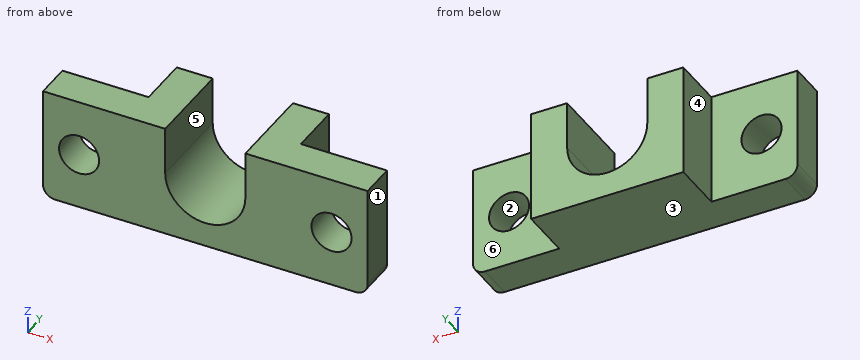
from build123d import *

# Parameters (mm, degrees)
SKETCH_1_W          = 81
SKETCH_1_H          = 28
EXTRUDE_1_DEPTH     = 9
SKETCH_2_W          = 38
SKETCH_2_H          = 28
EXTRUDE_2_DEPTH     = 13
CUT_EXTRUDE_1_DEPTH = 33
SKETCH_4_R          = 5
CUT_EXTRUDE_2_DEPTH = 33
SKETCH_5_R          = 5
CUT_EXTRUDE_3_DEPTH = 33
FILLET_1_R          = 3


with BuildPart() as part:
    # 스케치1 → 보스-돌출1 (new body)
    with BuildSketch(Plane(origin=(0, 0, 0), x_dir=(1, 0, 0), z_dir=(0, 1, 0))):
        with Locations((40.5, 14)):
            Rectangle(SKETCH_1_W, SKETCH_1_H)
    extrude(amount=EXTRUDE_1_DEPTH)

    # 스케치2 → 보스-돌출2 (add)
    with BuildSketch(Plane(origin=(0, 9, 0), x_dir=(1, 0, 0), z_dir=(0, 1, 0))):
        with Locations((40.5, 14)):
            Rectangle(SKETCH_2_W, SKETCH_2_H)
    extrude(amount=EXTRUDE_2_DEPTH)

    # 스케치3 → 컷-돌출1 (cut)
    with BuildSketch(Plane(origin=(0, 22, 0), x_dir=(1, 0, 0), z_dir=(0, 1, 0))):
        with BuildLine():
            Line((30.5, 0), (30.5, 11.914888689))
            ThreePointArc((30.5, 11.914888689), (40.5, 21.914888689), (50.5, 11.914888689))
            Line((50.5, 11.914888689), (50.5, 0))
            Line((50.5, 0), (30.5, 0))
        make_face()
    extrude(amount=-CUT_EXTRUDE_1_DEPTH, mode=Mode.SUBTRACT)

    # 스케치4 → 컷-돌출2 (cut)
    with BuildSketch(Plane(origin=(0, 9, 0), x_dir=(1, 0, 0), z_dir=(0, 1, 0))):
        with Locations(Location((9, 14, 0), (0, 0, 270))):
            Circle(SKETCH_4_R)
    extrude(amount=-CUT_EXTRUDE_2_DEPTH, mode=Mode.SUBTRACT)

    # 스케치5 → 컷-돌출3 (cut)
    with BuildSketch(Plane(origin=(0, 9, 0), x_dir=(1, 0, 0), z_dir=(0, 1, 0))):
        with Locations(Location((72, 14, 0), (0, 0, 270))):
            Circle(SKETCH_5_R)
    extrude(amount=-CUT_EXTRUDE_3_DEPTH, mode=Mode.SUBTRACT)

    # 필렛1
    fillet_1_edges = [part.edges().sort_by_distance(p)[0] for p in [
        (0, 4.5, -28),
        (81, 4.5, -28),
    ]]
    fillet(fillet_1_edges, radius=FILLET_1_R)


solid = part.part
Verification items for the finished model (mm, model axes). Face numbers are marked on the shaded views. A direction names the side the tool comes from. Give positions to 0.01 mm unless a question says otherwise; leave off trailing zeros. Write each loop counter-clockwise with the first axis right and the second up, starting at its lowest first coordinate (ties: lowest second). Pieces come first, ordered by that corner, then holes. Notation, with made-up numbers: (-17, 64.25) - (19, 64.25) arc R30 cw to (19, 89.25) - close; hole circle Ø7 at (71.5, 15). An arc over 180 degrees is marked (long way). Answer as CSV lines item,"result". Start each with the question number.
1. Thickness scan on line 1 (X direction, y = 7, z = -14); line 2 (Y direction, x = 15.5, z = -8); line 3 (X direction, y = 21.25, z = -8.25). Record the ranges inside material, lowest first.
2. Sectioned sample at C-C (z = -14). Record the boundary of the cut face in (x, y).
3. Sectioned sample at B-B (y = 3.25). Record the boundary of the cut face in (x, z).
4. Depth check by flat-ended pin: pin 1 (13 mm diameter, centred on y = 16.5, z = -8, fed in from +X); pin 2 (12 mm diameter, centred on x = 43, y = 15.5, fed in from +Z); pin 3 (4 mm diameter, centred on y = 15, z = -9.5, fed in from -X). Enter the tip coordinate at first touch or a pass-through.
5. Set-up check for the marked faces 4, 5 and 6: record each of +Z, -Z, +X, -X, +Y, -Y from which the full face is reachable in a straight line by a thin tool's end or side.
6. Sectioned sample at D-D (z = -5.5). Record the boundary of the cut face in (x, y), then the cut area to 3 significant figures.
7. Sectioned sample at A-A (x = 72). Record the boundary of the cut face in (y, z), then the cut area to 3 significant figures.
8. Draft check along X on the marked faces 1, 2 and 3. Enter one of: pulls with the +X half, pulls with the -X half, needs draft (parallel to the pull), parting line crosses it, or undercut.
Derived:
1,line 1,"0 to 4, 14 to 30.72, 50.28 to 67, 77 to 81"
1,line 2,"0 to 9"
1,line 3,"21.5 to 30.5, 50.5 to 59.5"
2,outline,"(0, 0) - (4, 0) - (4, 9) - (0, 9) - close; (14, 0) - (30.72, 0) - (30.72, 22) - (21.5, 22) - (21.5, 9) - (14, 9) - close; (50.28, 0) - (67, 0) - (67, 9) - (59.5, 9) - (59.5, 22) - (50.28, 22) - close; (77, 0) - (81, 0) - (81, 9) - (77, 9) - close"
3,outline,"(0, -25) arc R3 ccw to (3, -28) - (78, -28) arc R3 ccw to (81, -25) - (81, 0) - (50.5, 0) - (50.5, -11.91) arc R10 cw to (30.5, -11.91) - (30.5, 0) - (0, 0) - close; hole circle Ø10 at (9, -14); hole circle Ø10 at (72, -14)"
4,pin 1,"x = 59.5"
4,pin 2,"z = -17.18"
4,pin 3,"x = 21.5"
5,face 4,"+Z, -Z, -X, +Y"
5,face 5,"+Z, +Y, -Y"
5,face 6,"+Z, -Z, +X, +Y"
6,outline,"(0, 0) - (30.5, 0) - (30.5, 22) - (21.5, 22) - (21.5, 9) - (0, 9) - close; (50.5, 0) - (81, 0) - (81, 9) - (59.5, 9) - (59.5, 22) - (50.5, 22) - close"
6,area,"783 mm²"
7,outline,"(0, -28) - (9, -28) - (9, -19) - (0, -19) - close; (0, -9) - (9, -9) - (9, 0) - (0, 0) - close"
7,area,"162 mm²"
8,face 1,"pulls with the +X half"
8,face 2,"undercut"
8,face 3,"needs draft"
